Source: CAD feature listing. Evaluate the final solid. Frame: model axes, mm. Face numbers are marked on the shaded views. A direction names the side the tool comes from. Coordinates: 2 decimals unless noted, no trailing zeros. Order: outer loops, then holes, each group sorted by start corner. A loop starts at its lowest first (then second) coordinate and runs counter-clockwise, first axis right, second up.
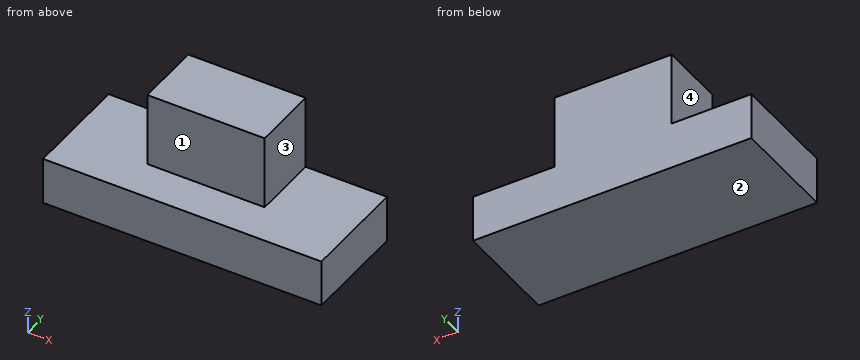
```python
from build123d import *

# Parameters (mm, degrees)
F0_W     = 131.7625
F0_H     = 50.8
F1_DEPTH = 22.225
F3_DEPTH = 34.925


with BuildPart() as f1:
    # F0 (on Top) → F1 (new body)
    with BuildSketch(Plane.XY):
        with Locations((65.88125, -25.4)):
            Rectangle(F0_W, F0_H)
    extrude(amount=F1_DEPTH)

    # F2 (on face) → F3 (join)
    with BuildSketch(Plane.XY.offset(22.225)):
        Polygon((93.271066, 0), (37.708566, 0), (37.708566, -25.4), (37.708566, -31.75), (93.271066, -31.75), align=None)
    extrude(amount=F3_DEPTH)


solid = f1.part
```
Q1. Pin query (flat end, axial travel): P1, Ø5, axis at x = 88, z = 28, coming from the -Y side; P2, Ø3, axis at y = -9.5, z = 42, coming from the +X side. Return the tip coordinate at first contact, or that it passes through.
Solutions:
P1: stops at y = -31.75
P2: stops at x = 93.27
Q2. Section query D-D on x = 59.5. Output: boundary loops of the cut face in (y, z) (3 decimals), plus the area to 3 significant figures.
Solutions:
outline: (-50.8, 0) - (0, 0) - (0, 57.15) - (-31.75, 57.15) - (-31.75, 22.225) - (-50.8, 22.225) - close
area: 2,240 mm2
Q3. Set-up query: the marked faces 1, 2, 3 and 4. Return all of +Z, -Z, +X, -X, +Y, -Y with unobstructed straight access to the full face (end or side cutting, diameter ignored); none if empty.
Solutions:
face 1: +Z, +X, -X, -Y
face 2: -Z, +X, -X, +Y, -Y
face 3: +Z, +X, +Y, -Y
face 4: +Z, -X, +Y, -Y
Q4. Material intervals for line 1 along X through (y, z) = (-24, 31.5); line 2 along Z through (x, y) = (126, -9) (3 decimals); line 3 along Y through (x, z) = (75, 35), sorted ascending.
Solutions:
line 1: x = 37.71 to 93.27
line 2: z = 0 to 22.225
line 3: y = -31.75 to 0
Q5. Section query C-C on z = 33.5. Output: boundary loops of the cut face in (x, y).
Solutions:
outline: (37.71, -31.75) - (93.27, -31.75) - (93.27, 0) - (37.71, 0) - close
Q6. Section query B-B on x = 122. Output: boundary loops of the cut face in (y, z) (3 decimals), plus the area to 3 significant figures.
Solutions:
outline: (-50.8, 0) - (0, 0) - (0, 22.225) - (-50.8, 22.225) - close
area: 1,130 mm2
